Source: CAD feature listing. Evaluate the final solid. Frame: model axes, mm. A direction names the side the tool comes from. Give positions to 0.01 mm unless a question says otherwise; leave off trailing zeros. Order: outer loops, then holes, each group sorted by start corner. A loop starts at its lowest first (then second) coordinate and runs counter-clockwise, first axis right, second up.
```python
from build123d import *

# Parameters (mm, degrees)
SKETCH2_R           = 1
BOSS_EXTRUDE1_DEPTH = 3


with BuildPart() as part:
    # Sketch2 → Boss-Extrude1 (new body)
    with BuildSketch(Plane(origin=(0, 0, 0), x_dir=(0, 0, -1), z_dir=(1, 0, 0))):
        with BuildLine():
            Line((19.216665357, -6.109306765), (15, -6.109306765))
            Line((15, -6.109306765), (0, 0))
            Line((0, 0), (-10.001460368, 0))
            ThreePointArc((-10.001460368, 0), (-12.001460368, -2), (-10.001460368, -4))
            Line((-10.001460368, -4), (-0.783334643, -4))
            Line((-0.783334643, -4), (14.216665357, -10.109306765))
            Line((14.216665357, -10.109306765), (19.216665357, -10.109306765))
            ThreePointArc((19.216665357, -10.109306765), (21.216665357, -8.109306765), (19.216665357, -6.109306765))
        make_face()
        with Locations((19.216665357, -8.109306765)):
            Circle(SKETCH2_R, mode=Mode.SUBTRACT)
        with Locations((-10.001460368, -2)):
            Circle(SKETCH2_R, mode=Mode.SUBTRACT)
    extrude(amount=BOSS_EXTRUDE1_DEPTH)


solid = part.part
```
1) Reachability of faces 5 (the flat face through (3, -5, -5)), 6 (the flat face through (1, -6.109, -17)), 7 (the flat face through (1, -4, 5)) from +Z, -Z, +X, -X, +Y, -Y: full face, straight path, thin tool, end or side. Return the list, or none.
Report:
face 5: +Z, -Z, +X, +Y, -Y
face 6: -Z, +X, -X, +Y
face 7: +Z, +X, -X, -Y
2) Section query B-B, the plane y = -2. Return the cut outline in (x, z).
Report:
outline: (0, -4.91) - (3, -4.91) - (3, 9) - (0, 9) - close; (0, 11) - (3, 11) - (3, 12) - (0, 12) - close
3) Pin query (flat end, axial travel): pin 1 (1 mm diameter, centred on x = 2.5, z = -13.5, fed in from +Y). Return the tip coordinate at first contact, or that it passes through.
Report:
pin 1: stops at y = -5.29
4) Section query C-C, the plane z = -17.5. Return the cut outline in (x, y), and give its area (3 significant figures).
Report:
outline: (0, -10.11) - (3, -10.11) - (3, -6.11) - (0, -6.11) - close
area: 12.0 mm2
5) Section query D-D, the plane y = -4.75. Return the cut outline in (x, z), and give its area (3 significant figures).
Report:
outline: (0, -11.66) - (3, -11.66) - (3, -1.06) - (0, -1.06) - close
area: 31.8 mm2
6) Section query A-A, the plane x = 1.85. Return the cut outline in (y, z), and give its area (3 significant figures).
Report:
outline: (-10.11, -19.22) arc R2 ccw to (-6.11, -19.22) - (-6.11, -15) - (0, 0) - (0, 10) arc R2 ccw to (-4, 10) - (-4, 0.78) - (-10.11, -14.22) - close; hole circle Ø2 at (-8.11, -19.22); hole circle Ø2 at (-2, 10)
area: 128 mm2
7) Draft query along Y for faces 1 (the cylindrical face through (1, -2, 12)), 2 (the flat face through (1, 0, 5)), 3 (the cylindrical face through (1.48, -7.81, -20.17)), 4 (the cylindrical face through (1, -2, 9)). Return one class per face: +Y half, -Y half, draft (parallel to the pull), parting line (faces both ways), or undercut.
Report:
face 1: parting line
face 2: +Y half
face 3: undercut
face 4: undercut
8) Material intervals for L1, parallel to Y at x = 2.9, z = 3; L2, parallel to Y at x = 0.4, z = -19; L3, parallel to Z at x = 1.5, y = -7.25, sorted ascending.
Report:
L1: y = -4 to 0
L2: y = -10.11 to -9.09, -7.13 to -6.11
L3: z = -21.02 to -19.73, -18.71 to -7.2
